from build123d import *

# Parameters (mm, degrees)
F1_DEPTH = 150
F2_W     = 34.5892625776
F2_H     = 120
F3_DEPTH = 25
F4_R     = 4.99999


# Not quite as in the source:
# - a fillet or chamfer is up to 0.001 mm smaller than in the source, because OpenCascade refuses the exact size


with BuildPart() as f1:
    # F0 (on Top) → F1 (new body)
    with BuildSketch(Plane.XY):
        Polygon((-17, 31.4391109618), (-22, 31.4391109618), (-22, -10), (-17, -10), (-17, 0), (0, 0), (0, -20), (4.7985620563, -20), (4.7985620563, 0), (11, 0), (11, 31.4391109618), (6, 31.4391109618), (6, 16.4391109618), (-17, 16.4391109618), align=None)
    extrude(amount=F1_DEPTH)

    # F2 (on Right) → F3 (cut)
    with BuildSketch(Plane.YZ):
        with Locations((38.7337422506, 75)):
            Rectangle(F2_W, F2_H)
    extrude(amount=-F3_DEPTH, mode=Mode.SUBTRACT)

    # F4 (radius 5 in the source; OpenCascade refuses exactly that, so slightly less here)
    f4_edges = [f1.edges().sort_by_distance(p)[0] for p in [
        (-19.5, 21.439111, 135),
        (-19.5, 31.439111, 135),
        (-19.5, 21.439111, 15),
        (-19.5, 31.439111, 15),
        (-19.5, 31.439111, 150),
        (-19.5, -10, 150),
        (-19.5, 31.439111, 0),
        (-19.5, -10, 0),
        (-22, 10.719555, 0),
        (-22, -10, 75),
        (-22, 10.719555, 150),
        (-22, 31.439111, 142.5),
        (-22, 26.439111, 135),
        (-22, 21.439111, 75),
        (-22, 26.439111, 15),
        (-22, 31.439111, 7.5),
    ]]
    fillet(f4_edges, radius=F4_R)


solid = f1.part
Work out the finished part from the listing and answer in its coordinate system (mm). A direction names the side the tool comes from. Give positions to 0.01 mm unless a question says otherwise; leave off trailing zeros. Write each loop counter-clockwise with the first axis right and the second up, starting at its lowest first coordinate (ties: lowest second). Pieces come first, ordered by that corner, then holes. Notation, with made-up numbers: (16.5, 22.25) - (72.5, 22.25) arc R28 cw to (72.5, 51.25) - close; hole circle Ø10 at (79, -25). An arc over 180 degrees is marked (long way). One line per item, written item: value. Start each with the question number.
1. Find section B-B (x = -10.5). Write down the section's boundary in (y, z), then the cut area to 3 significant figures.
2. Find section D-D (y = -11.5). Write down the section's boundary in (x, z), then the cut area to 3 significant figures.
3. For faces 1 (the flat face through (0, -10, 74)), 2 (the flat face through (-5, 16.439, 74)), 3 (the flat face through (4.799, -10, 74)), determine the directions among +Z, -Z, +X, -X, +Y, -Y from which every point of the face is accessible in a straight line to the end or side of a thin tool.
4. Consider probe 1 along Y at (x, z) = (-5.5, 132); probe 2 along Y at (x, z) = (3, 41); probe 3 along X at (y, z) = (-8.5, 13). Determine where each line is inside the solid, lowest interval first.
5. Find section C-C (y = 24). State how many separate pieces and enclosed holes the cut face has, then the cut area to 3 significant figures.
6. Given pin 1 (11.5 mm diameter, centred on x = -10.5, z = 43, fed in from +Y); pin 2 (4 mm diameter, centred on x = -17.5, z = 60, fed in from -Y); pin 3 (7.5 mm diameter, centred on y = 23, z = 81, fed in from -X), each flat-ended and moving along its own axis, determine where each tip first touches the part or whether it passes through.
7. For a pull along Z with two mould halves and no side action, classify faces 4 (the flat face through (-17, 21, 74)), 5 (the flat face through (0, 6, 150)), 6 (the cylindrical face through (-20.57, 19.94, 75.77)) as +Z half, -Z half, draft (parallel to the pull), parting line (faces both ways), or undercut.
Geometry results:
1. outline: (0, 0) - (16.44, 0) - (16.44, 150) - (0, 150) - close
1. area: 2,470 mm2
2. outline: (0, 0) - (4.8, 0) - (4.8, 150) - (0, 150) - close
2. area: 720 mm2
3. face 1: +Z, -Z, -Y
3. face 2: +Z, -Z, +Y
3. face 3: +Z, -Z, +X, -Y
4. probe 1: 0 to 16.44
4. probe 2: -20 to 16.44
4. probe 3: -20.57 to -17, 0 to 4.8
5. separate pieces: 3
5. enclosed holes: 0
5. area: 884 mm2
6. pin 1: y = 16.44
6. pin 2: y = -10
6. pin 3: x = -21.14
7. face 4: draft
7. face 5: +Z half
7. face 6: undercut
